from build123d import *

# Parameters (mm, degrees)
SCHIZZO1_R                   = 15
ESTRUSIONE_ESTRUSIONE1_DEPTH = 50
SCHIZZO2_W                   = 50
SCHIZZO2_H                   = 230
ESTRUSIONE_ESTRUSIONE2_DEPTH = 40
SCHIZZO3_W                   = 130
SCHIZZO3_H                   = 180
TAGLIO_ESTRUSIONE1_DEPTH     = 423.621427401


with BuildPart() as part:
    # Schizzo1 → Estrusione-Estrusione1 (new, symmetric)
    with BuildSketch(Plane.XY):
        with BuildLine():
            Line((25, 384.888851883), (25, -15.111148117))
            ThreePointArc((25, -15.111148117), (0, -40.111148117), (-25, -15.111148117))
            Line((-25, -15.111148117), (-25, 384.888851883))
            ThreePointArc((-25, 384.888851883), (0, 409.888851883), (25, 384.888851883))
        make_face()
        with Locations((0, 384.888851883)):
            Circle(SCHIZZO1_R, mode=Mode.SUBTRACT)
        with Locations((0, -15.111148117)):
            Circle(SCHIZZO1_R, mode=Mode.SUBTRACT)
    extrude(amount=ESTRUSIONE_ESTRUSIONE1_DEPTH, both=True)

    # Schizzo2 → Estrusione-Estrusione2 (add)
    with BuildSketch(Plane.XY.offset(50)):
        with Locations((0, 179.888851883)):
            Rectangle(SCHIZZO2_W, SCHIZZO2_H)
    estrusione_estrusione2 = extrude(amount=ESTRUSIONE_ESTRUSIONE2_DEPTH)

    # Specchia1: Estrusione-Estrusione2 across plane
    add(estrusione_estrusione2.mirror(Plane.XY))

    # Schizzo3 → Taglio-Estrusione1 (cut, through all)
    with BuildSketch(Plane(origin=(25, 0, 0), x_dir=(0, 0, -1), z_dir=(1, 0, 0))):
        with Locations((0, 179.888851883)):
            Rectangle(SCHIZZO3_W, SCHIZZO3_H)
    extrude(amount=-TAGLIO_ESTRUSIONE1_DEPTH, mode=Mode.SUBTRACT)


solid = part.part
For this review, take the finished solid that the model builds, in its own axes (mm). A direction names the side the tool comes from. Round coordinates to 2 decimals unless told otherwise and drop trailing zeros. Loops run counter-clockwise (first coordinate to the right, second up) from the corner with the lowest first, then second, coordinate; pieces in that order, holes last. Notation, with made-up numbers: (14.25, -27) - (69.25, -27) arc R19 cw to (69.25, -13) - close; hole circle Ø5 at (42.5, 43). An arc over 180 degrees is marked (long way). Use one line per item in the form item = value.
1) We need section C-C on x = 0. Write out the cut boundary in (y, z).
Solutions:
outline = (-40.11, -50) - (-30.11, -50) - (-30.11, 50) - (-40.11, 50) - close; (-0.11, -50) - (64.89, -50) - (64.89, -90) - (294.89, -90) - (294.89, -50) - (369.89, -50) - (369.89, 50) - (294.89, 50) - (294.89, 90) - (64.89, 90) - (64.89, 50) - (-0.11, 50) - close; (399.89, -50) - (409.89, -50) - (409.89, 50) - (399.89, 50) - close; hole (89.89, -65) - (269.89, -65) - (269.89, 65) - (89.89, 65) - close
2) Wall thickness on probe 1 along Y at (x, z) = (0, -28); probe 2 along Y at (x, z) = (5, -40); probe 3 along Z at (x, y) = (-2, 262): over which ranges is each line inside the solid? List them lowest first.
Solutions:
probe_1 = -40.11 to -30.11, -0.11 to 89.89, 269.89 to 369.89, 399.89 to 409.89
probe_2 = -39.61 to -29.25, -0.97 to 89.89, 269.89 to 370.75, 399.03 to 409.38
probe_3 = -90 to -65, 65 to 90
3) We need section B-B on y = 174. Write out the cut boundary in (x, z), then the cut area to 3 significant figures.
Solutions:
outline = (-25, -90) - (25, -90) - (25, -65) - (-25, -65) - close; (-25, 65) - (25, 65) - (25, 90) - (-25, 90) - close
area = 2,500 mm2
4) We need section D-D on x = 19.5. Write out the cut boundary in (y, z), then the cut area to 3 significant figures.
Solutions:
outline = (-30.76, -50) - (64.89, -50) - (64.89, -90) - (294.89, -90) - (294.89, -50) - (400.53, -50) - (400.53, 50) - (294.89, 50) - (294.89, 90) - (64.89, 90) - (64.89, 50) - (-30.76, 50) - close; hole (89.89, -65) - (269.89, -65) - (269.89, 65) - (89.89, 65) - close
area = 38,100 mm2
5) Mouldability with a two-part tool opening along Z and no side actions: class faces 1 (the face through (0, 179, 65)), 2 (the face through (0, 181, 90)), 3 (the face through (-25, 271, 1)) as pulls with the +Z half, pulls with the -Z half, needs draft (parallel to the pull), parting line crosses it, or undercut.
Solutions:
face_1 = undercut
face_2 = pulls with the +Z half
face_3 = needs draft
6) We need section A-A on z = -43. Write out the cut boundary in (x, y), then the cut area to 3 significant figures.
Solutions:
outline = (-25, -15.11) arc R25 ccw to (25, -15.11) - (25, 89.89) - (-25, 89.89) - close; (-25, 269.89) - (25, 269.89) - (25, 384.89) arc R25 ccw to (-25, 384.89) - close; hole circle Ø30 at (0, -15.11); hole circle Ø30 at (0, 384.89)
area = 11,500 mm2
7) Clearance check with flat-ended pins moving along their axes: P1, Ø1.5, axis at x = 2.5, z = -55, coming from the -Y side; P2, Ø24, axis at x = 0, y = 384.89, coming from the -Z side; P3, Ø1, axis at x = 11, z = 40, coming from the -Y side; P4, Ø1, axis at x = -15, z = 67.5, coming from the +Y side. State where each tip first meets the part, or that it passes through.
Solutions:
P1 = 64.89
P2 = through
P3 = -37.8
P4 = 294.89
8) Tool access review of faces 4 (the face through (0, 269.889, 1)), 5 (the face through (0, 294.889, 70)), 6 (the face through (0, 64.889, 70)), 7 (the face through (0, 64.889, -70)): name each direction out of +Z, -Z, +X, -X, +Y, -Y from which nothing blocks a thin tool from reaching the whole face with its end or side.
Solutions:
face_4 = +X, -X
face_5 = +Z, +X, -X, +Y
face_6 = +Z, +X, -X, -Y
face_7 = -Z, +X, -X, -Y
